Geometry: final body of the model. Coordinates: model frame, mm. A direction names the side the tool comes from. Give positions to 0.01 mm unless a question says otherwise; leave off trailing zeros. Loops run counter-clockwise (first coordinate to the right, second up) from the corner with the lowest first, then second, coordinate; pieces in that order, holes last.
from build123d import *

# Parameters (mm, degrees)
ESQUISSE1_W             = 57.15
ESQUISSE1_H             = 57.15
BOSS_EXTRU_1_DEPTH      = 43.942
ENL_V_MAT_EXTRU_1_DEPTH = 38.862
ENL_V_MAT_EXTRU_2_DEPTH = 38.862
ENL_V_MAT_EXTRU_3_DEPTH = 38.862
ENL_V_MAT_EXTRU_4_DEPTH = 38.862
ENL_V_MAT_EXTRU_5_DEPTH = 38.862
ENL_V_MAT_EXTRU_6_DEPTH = 38.862
ENL_V_MAT_EXTRU_7_DEPTH = 38.862
ENL_V_MAT_EXTRU_8_DEPTH = 38.862
ESQUISSE10_R            = 19.05
BOSS_EXTRU_2_DEPTH      = 1.524
ESQUISSE11_R            = 3.175
BOSS_EXTRU_3_DEPTH      = 19.05
ENL_V_MAT_EXTRU_9_DEPTH = 14.986
ESQUISSE13_W            = 0.635
ESQUISSE13_H            = 85.725
ESQUISSE14_W            = 0.635
ESQUISSE14_H            = 85.725
ESQUISSE15_W            = 0.635
ESQUISSE15_H            = 85.725
ESQUISSE16_W            = 0.635
ESQUISSE16_H            = 85.725
PER_AGE1_D              = 5.08
PER_AGE1_DEPTH          = 25.654
CHANFREIN1_SIZE         = 0.254
CONG_1_R                = 2.54


with BuildPart() as part:
    # Esquisse1 → Boss.-Extru.1 (new body)
    with BuildSketch(Plane.XY.offset(43.942)):
        Rectangle(ESQUISSE1_W, ESQUISSE1_H)
    extrude(amount=-BOSS_EXTRU_1_DEPTH)

    # Esquisse2 → Enlèv. mat.-Extru.1 (cut)
    with BuildSketch(Plane(origin=(0, 0, 0), x_dir=(-1, 0, 0), z_dir=(0, 0, -1))):
        with BuildLine():
            Line((-28.575, -28.575), (-14.692533342, -28.575))
            ThreePointArc((-14.692533342, -28.575), (-22.720047986, -22.720047986), (-28.575, -14.692533342))
            Line((-28.575, -14.692533342), (-28.575, -28.575))
        make_face()
    extrude(amount=-ENL_V_MAT_EXTRU_1_DEPTH, mode=Mode.SUBTRACT)

    # Esquisse3 → Enlèv. mat.-Extru.2 (cut)
    with BuildSketch(Plane(origin=(0, 0, 0), x_dir=(-1, 0, 0), z_dir=(0, 0, -1))):
        with BuildLine():
            Line((-19.2786, -25.7048), (-19.2786, -19.2786))
            Line((-19.2786, -19.2786), (-25.7048, -19.2786))
            ThreePointArc((-25.7048, -19.2786), (-22.720047986, -22.720047986), (-19.2786, -25.7048))
        make_face()
    extrude(amount=-ENL_V_MAT_EXTRU_2_DEPTH, mode=Mode.SUBTRACT)

    # Esquisse4 → Enlèv. mat.-Extru.3 (cut)
    with BuildSketch(Plane(origin=(0, 0, 0), x_dir=(-1, 0, 0), z_dir=(0, 0, -1))):
        with BuildLine():
            Line((-28.575, 28.575), (-28.575, 14.692533342))
            ThreePointArc((-28.575, 14.692533342), (-22.720047986, 22.720047986), (-14.692533342, 28.575))
            Line((-14.692533342, 28.575), (-28.575, 28.575))
        make_face()
    extrude(amount=-ENL_V_MAT_EXTRU_3_DEPTH, mode=Mode.SUBTRACT)

    # Esquisse5 → Enlèv. mat.-Extru.4 (cut)
    with BuildSketch(Plane(origin=(0, 0, 0), x_dir=(-1, 0, 0), z_dir=(0, 0, -1))):
        with BuildLine():
            Line((-25.7048, 19.2786), (-19.2786, 19.2786))
            Line((-19.2786, 19.2786), (-19.2786, 25.7048))
            ThreePointArc((-19.2786, 25.7048), (-22.720047986, 22.720047986), (-25.7048, 19.2786))
        make_face()
    extrude(amount=-ENL_V_MAT_EXTRU_4_DEPTH, mode=Mode.SUBTRACT)

    # Esquisse6 → Enlèv. mat.-Extru.5 (cut)
    with BuildSketch(Plane(origin=(0, 0, 0), x_dir=(-1, 0, 0), z_dir=(0, 0, -1))):
        with BuildLine():
            Line((28.575, 28.575), (14.692533342, 28.575))
            ThreePointArc((14.692533342, 28.575), (22.720047986, 22.720047986), (28.575, 14.692533342))
            Line((28.575, 14.692533342), (28.575, 28.575))
        make_face()
    extrude(amount=-ENL_V_MAT_EXTRU_5_DEPTH, mode=Mode.SUBTRACT)

    # Esquisse7 → Enlèv. mat.-Extru.6 (cut)
    with BuildSketch(Plane(origin=(0, 0, 0), x_dir=(-1, 0, 0), z_dir=(0, 0, -1))):
        with BuildLine():
            Line((19.2786, 25.7048), (19.2786, 19.2786))
            Line((19.2786, 19.2786), (25.7048, 19.2786))
            ThreePointArc((25.7048, 19.2786), (22.720047986, 22.720047986), (19.2786, 25.7048))
        make_face()
    extrude(amount=-ENL_V_MAT_EXTRU_6_DEPTH, mode=Mode.SUBTRACT)

    # Esquisse8 → Enlèv. mat.-Extru.7 (cut)
    with BuildSketch(Plane(origin=(0, 0, 0), x_dir=(-1, 0, 0), z_dir=(0, 0, -1))):
        with BuildLine():
            Line((28.575, -28.575), (28.575, -14.692533342))
            ThreePointArc((28.575, -14.692533342), (22.720047986, -22.720047986), (14.692533342, -28.575))
            Line((14.692533342, -28.575), (28.575, -28.575))
        make_face()
    extrude(amount=-ENL_V_MAT_EXTRU_7_DEPTH, mode=Mode.SUBTRACT)

    # Esquisse9 → Enlèv. mat.-Extru.8 (cut)
    with BuildSketch(Plane(origin=(0, 0, 0), x_dir=(-1, 0, 0), z_dir=(0, 0, -1))):
        with BuildLine():
            Line((25.7048, -19.2786), (19.2786, -19.2786))
            Line((19.2786, -19.2786), (19.2786, -25.7048))
            ThreePointArc((19.2786, -25.7048), (22.720047986, -22.720047986), (25.7048, -19.2786))
        make_face()
    extrude(amount=-ENL_V_MAT_EXTRU_8_DEPTH, mode=Mode.SUBTRACT)

    # Esquisse10 → Boss.-Extru.2 (add)
    with BuildSketch(Plane.XY.offset(43.942)):
        Circle(ESQUISSE10_R)
    extrude(amount=BOSS_EXTRU_2_DEPTH)

    # Esquisse11 → Boss.-Extru.3 (add)
    with BuildSketch(Plane.XY.offset(45.466)):
        Circle(ESQUISSE11_R)
    extrude(amount=BOSS_EXTRU_3_DEPTH)

    # Esquisse12 → Enlèv. mat.-Extru.9 (cut)
    with BuildSketch(Plane.XY.offset(64.516)):
        with BuildLine():
            Line((-1.722711816, 2.667), (1.722711816, 2.667))
            ThreePointArc((1.722711816, 2.667), (0, 3.175), (-1.722711816, 2.667))
        make_face()
    extrude(amount=-ENL_V_MAT_EXTRU_9_DEPTH, mode=Mode.SUBTRACT)

    # Esquisse13 → Révolution1 (revolve)
    with BuildSketch(Plane(origin=(0, 0, 12.7), x_dir=(-1, 0, 0), z_dir=(0, 0, -1))):
        with Locations((1.7145, 71.4375)):
            Rectangle(ESQUISSE13_W, ESQUISSE13_H)
    revolve(axis=Axis((-2.032, 28.575, 12.7), (0, 1, 0)))

    # Esquisse14 → Révolution2 (revolve)
    with BuildSketch(Plane(origin=(0, 0, 12.7), x_dir=(-1, 0, 0), z_dir=(0, 0, -1))):
        with Locations((-2.3495, 71.4375)):
            Rectangle(ESQUISSE14_W, ESQUISSE14_H)
    revolve(axis=Axis((2.032, 28.575, 12.7), (0, 1, 0)))

    # Esquisse15 → Révolution3 (revolve)
    with BuildSketch(Plane(origin=(0, 0, 14.732), x_dir=(-1, 0, 0), z_dir=(0, 0, -1))):
        with Locations((-0.3175, 71.4375)):
            Rectangle(ESQUISSE15_W, ESQUISSE15_H)
    revolve(axis=Axis((0, 28.575, 14.732), (0, 1, 0)))

    # Esquisse16 → Révolution4 (revolve)
    with BuildSketch(Plane(origin=(0, 0, 10.668), x_dir=(-1, 0, 0), z_dir=(0, 0, -1))):
        with Locations((-0.3175, 71.4375)):
            Rectangle(ESQUISSE16_W, ESQUISSE16_H)
    revolve(axis=Axis((0, 28.575, 10.668), (0, 1, 0)))

    # Perçage1
    with Locations(Plane(origin=(0, 0, 38.862), x_dir=(-1, 0, 0), z_dir=(0, 0, -1))):
        with Locations((-23.622, -23.622), (-23.622, 23.622), (23.622, 23.622), (23.622, -23.622)):
            Hole(PER_AGE1_D / 2, depth=PER_AGE1_DEPTH)

    # Chanfrein1
    chanfrein1_edges = [part.edges().sort_by_distance(p)[0] for p in [
        (-1.51838977, -2.78838977, 64.516),
    ]]
    chamfer(chanfrein1_edges, length=CHANFREIN1_SIZE)

    # Congé1
    cong_1_edges = [part.edges().sort_by_distance(p)[0] for p in [
        (-19.2786, -19.2786, 19.431),
        (28.575, -28.575, 41.402),
        (19.2786, -19.2786, 19.431),
        (28.575, 28.575, 41.402),
        (19.2786, 19.2786, 19.431),
        (-28.575, 28.575, 41.402),
        (-19.2786, 19.2786, 19.431),
        (-28.575, -28.575, 41.402),
    ]]
    fillet(cong_1_edges, radius=CONG_1_R)


solid = part.part
Item 1: Section query B-B on z = 19. Return loops of the section in (x, y) (3 decimals).
Values follow:
outline: (-28.575, -14.693) arc R32.131 ccw to (-25.705, -19.279) - (-21.819, -19.279) arc R2.54 cw to (-19.279, -21.819) - (-19.279, -25.705) arc R32.131 ccw to (-14.693, -28.575) - (14.693, -28.575) arc R32.131 ccw to (19.279, -25.705) - (19.279, -21.819) arc R2.54 cw to (21.819, -19.279) - (25.705, -19.279) arc R32.131 ccw to (28.575, -14.693) - (28.575, 14.693) arc R32.131 ccw to (25.705, 19.279) - (21.819, 19.279) arc R2.54 cw to (19.279, 21.819) - (19.279, 25.705) arc R32.131 ccw to (14.693, 28.575) - (-14.693, 28.575) arc R32.131 ccw to (-19.279, 25.705) - (-19.279, 21.819) arc R2.54 cw to (-21.819, 19.279) - (-25.705, 19.279) arc R32.131 ccw to (-28.575, 14.693) - close
Item 2: Set-up query: faces 5 (the face through (20.003, -20.042, 19.703)), 6 (the face through (0, 2.667, 57)), 7 (the face through (23.3, 26.4, 38.862)), 8 (the face through (-23.1, 26.4, 38.862)). Return all of +Z, -Z, +X, -X, +Y, -Y with unobstructed straight access to the full face (end or side cutting, diameter ignored); none if empty.
Values follow:
face 5: -Z, +X, -Y
face 6: +Z, +X, -X, +Y
face 7: -Z, +X, +Y
face 8: -Z, -X, +Y
Item 3: Section query C-C on z = 41. Return loops of the section in (x, y) (3 decimals), plus the area to 3 significant figures.
Values follow:
outline: (-28.575, -26.035) arc R2.54 ccw to (-26.035, -28.575) - (26.035, -28.575) arc R2.54 ccw to (28.575, -26.035) - (28.575, 26.035) arc R2.54 ccw to (26.035, 28.575) - (-26.035, 28.575) arc R2.54 ccw to (-28.575, 26.035) - close; hole circle Ø5.08 at (-23.622, -23.622); hole circle Ø5.08 at (-23.622, 23.622); hole circle Ø5.08 at (23.622, -23.622); hole circle Ø5.08 at (23.622, 23.622)
area: 3,180 mm2
Item 4: Pin query (flat end, axial travel): pin 1 (4.5 mm diameter, centred on x = 24, z = 17.5, fed in from +Y); pin 2 (4 mm diameter, centred on y = 94.5, z = 7.5, fed in from +X); pin 3 (3 mm diameter, centred on y = 23, z = 19.5, fed in from +X); pin 4 (4.5 mm diameter, centred on x = 23, z = 14.5, fed in from -Y). Return the tip coordinate at first contact, or that it passes through.
Values follow:
pin 1: stops at y = 19.28
pin 2: passes through
pin 3: stops at x = 19.3
pin 4: stops at y = -19.51
Item 5: Draft query along Y for faces 1 (the face through (25.97, -24.59, 41.44)), 2 (the face through (24, 19.279, 19)), 3 (the face through (-24, -19.279, 19)), 4 (the face through (-25.494, 25.339, 41.438)). Return one class per face: +Y half, -Y half, draft (parallel to the pull), parting line (faces both ways), or undercut.
Values follow:
face 1: undercut
face 2: +Y half
face 3: -Y half
face 4: undercut
Item 6: Section query D-D on y = 50. Return loops of the section in (x, z) (3 decimals).
Values follow:
outline: circle Ø1.27 at (-2.032, 12.7); circle Ø1.27 at (0, 10.668); circle Ø1.27 at (0, 14.732); circle Ø1.27 at (2.032, 12.7)
Item 7: Section query A-A on y = 0. Return loops of the section in (x, z) (3 decimals).
Values follow:
outline: (-28.575, 0) - (28.575, 0) - (28.575, 43.942) - (19.05, 43.942) - (19.05, 45.466) - (3.175, 45.466) - (3.175, 64.262) - (2.921, 64.516) - (-2.921, 64.516) - (-3.175, 64.262) - (-3.175, 45.466) - (-19.05, 45.466) - (-19.05, 43.942) - (-28.575, 43.942) - close
Item 8: Ray query, probe 1 along Z at (x, y) = (-7, -7); probe 2 along Z at (x, y) = (-11, 16.5); probe 3 along Y at (x, z) = (-24, 33.5). Return the intervals inside material, ascending.
Values follow:
probe 1: z = 0 to 45.47
probe 2: z = 0 to 43.94
probe 3: y = -19.28 to 19.28
